Verification items for the finished model (mm, model axes). Round coordinates to 2 decimals unless told otherwise and drop trailing zeros. Order: outer loops, then holes, each group sorted by start corner. A loop starts at its lowest first (then second) coordinate and runs counter-clockwise, first axis right, second up. Notation, with made-up numbers: M 5,-21.5 L 22,-21.5 A31 cw 22,7.5 Z; hole C 56,27 d9. An arc over 180 degrees is marked long. Use CSV: the item, a comma, the result in double quotes. Start each with the question number.
Q1. Scan lines: line 1 (Y direction, x = 59, z = 0.45); line 2 (Y direction, x = 99.5, z = 0.3); line 3 (X direction, y = 33, z = 0.95). Record each from-to range of solid material in increasing order.
Q2. Sectioned sample at C-C (z = 0.65). State how many separate pieces and enclosed holes the cut face has, and give its area (3 significant figures).
Q3. Sectioned sample at A-A (x = 125). Enter the section's corners in (y, z).
Q4. Gauge pin test, flat ends, axial feed: pin 1 Ø0.5 at (x, z) = (147, 0.5) entering from +Y; pin 2 Ø2 at (x, y) = (21.21, 106.97) entering from -Z; pin 3 Ø0.5 at (x, z) = (164, 0.5) entering from +Y; pin 4 Ø0.5 at (x, z) = (102, 0.5) entering from +Y. Record the tip position at first contact, or that the pin passes through.
Q5. Sectioned sample at B-B (y = 61). Enter the section's corners in (x, z), and give its area (3 significant figures).
```python
from build123d import *
from build123d.topology import SkipClean

# Parameters (mm, degrees)
CROQUIS1_R              = 1.25
CROQUIS1_R_2            = 2.5
SALIENTE_EXTRUIR1_DEPTH = 1


with BuildPart() as part:
    # Croquis1 → Saliente-Extruir1 (new body)
    with BuildSketch(Plane.XY):
        with BuildLine():
            Line((64.278746094, 29.055249422), (61.278746094, 23.859096999))
            Line((61.278746094, 23.859096999), (67.340923921, 20.359096999))
            Line((67.340923921, 20.359096999), (85.5274574, 30.859096999))
            Line((85.5274574, 30.859096999), (112.5274574, 30.859096999))
            Line((112.5274574, 30.859096999), (112.5274574, 31.859096999))
            ThreePointArc((112.5274574, 31.859096999), (113.027457314, 32.359096999), (113.527457227, 31.859096999))
            Line((113.527457227, 31.859096999), (116.527457227, 31.859096999))
            ThreePointArc((116.527457227, 31.859096999), (117.027457227, 32.359096999), (117.527457227, 31.859096999))
            Line((117.527457227, 31.859096999), (117.527457227, 30.859096999))
            Line((117.527457227, 30.859096999), (144.527457227, 30.859096999))
            Line((144.527457227, 30.859096999), (162.713990707, 20.359096999))
            Line((162.713990707, 20.359096999), (174.83834636, 27.359096999))
            Line((174.83834636, 27.359096999), (174.83834636, 41.359096999))
            Line((174.83834636, 41.359096999), (167.83834636, 53.483452652))
            Line((167.83834636, 53.483452652), (158.83834636, 53.483452652))
            Line((158.83834636, 53.483452652), (148.446041514, 47.483452652))
            Line((148.446041514, 47.483452652), (145.446041514, 47.483452652))
            Line((145.446041514, 47.483452652), (143.946041514, 44.88537644))
            ThreePointArc((143.946041514, 44.88537644), (143.77192137, 44.012873167), (142.92105094, 44.272871814))
            Line((142.92105094, 44.272871814), (137.724898517, 47.272871814))
            Line((137.724898517, 47.272871814), (81.724898517, 47.272871814))
            Line((81.724898517, 47.272871814), (76.528746094, 50.272871814))
            Line((76.528746094, 50.272871814), (75.278746094, 48.107808305))
            ThreePointArc((75.278746094, 48.107808305), (76.193809604, 44.692744795), (72.778746094, 43.777681286))
            Line((72.778746094, 43.777681286), (71.778746094, 42.045630478))
            Line((71.778746094, 42.045630478), (72.428265147, 41.670630478))
            Line((72.428265147, 41.670630478), (64.928265147, 28.680249422))
            Line((64.928265147, 28.680249422), (64.278746094, 29.055249422))
        make_face()
        with Locations((76.571886424, 30.884748108)):
            Circle(CROQUIS1_R, mode=Mode.SUBTRACT)
        with Locations((153.286799356, 30.709365751)):
            Circle(CROQUIS1_R, mode=Mode.SUBTRACT)
        Polygon((166.425687586, 29.430249422), (165.776168533, 29.055249422), (165.12664948, 28.680249422), (157.62664948, 41.670630478), (158.276168533, 42.045630478), (158.925687586, 42.420630478), align=None, mode=Mode.SUBTRACT)
        Polygon((88.277457227, 42.272871814), (89.277457227, 43.272871814), (110.277457227, 43.272871814), (111.277457227, 42.272871814), (111.277457227, 37.272871814), (110.277457227, 36.272871814), (89.277457227, 36.272871814), (88.277457227, 37.272871814), align=None, mode=Mode.SUBTRACT)
        Polygon((119.277457227, 42.272871814), (120.277457227, 43.272871814), (133.277457227, 43.272871814), (134.277457227, 42.272871814), (134.277457227, 37.272871814), (133.277457227, 36.272871814), (120.277457227, 36.272871814), (119.277457227, 37.272871814), align=None, mode=Mode.SUBTRACT)
        with Locations((139.527457227, 41.32468677)):
            Circle(CROQUIS1_R, mode=Mode.SUBTRACT)
        with Locations((170.58834636, 40.698418571)):
            Circle(CROQUIS1_R, mode=Mode.SUBTRACT)
        with Locations((156.026168533, 45.942744795)):
            Circle(CROQUIS1_R_2, mode=Mode.SUBTRACT)
    saliente_extruir1 = extrude(amount=SALIENTE_EXTRUIR1_DEPTH)

    # Simetría2: Saliente-Extruir1 across plane
    with SkipClean():  # the faces are left unmerged after this step: merging them gives an invalid solid
        add(saliente_extruir1.mirror(Plane(origin=(35.627767514, -20.569701165, 1), x_dir=(0, 0, 1), z_dir=(0.8660254037844365, -0.5000000000000039, 0))))


solid = part.part
```
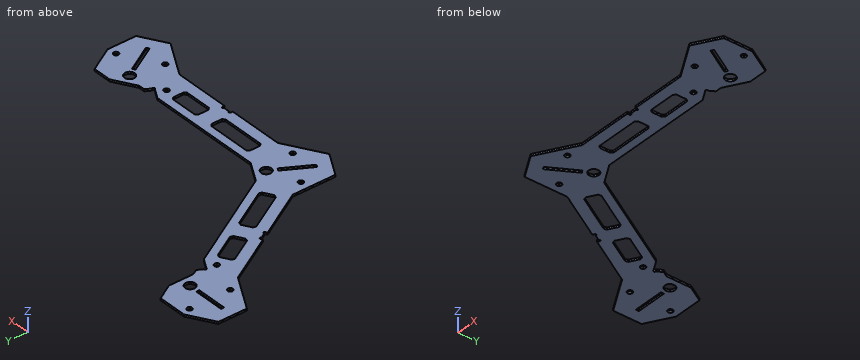
Verdict:
1,line 1,"y = 25.17 to 39.59, 41.64 to 54.05, 66.63 to 74.63"
1,line 2,"y = 30.86 to 36.27, 43.27 to 47.27"
1,line 3,"x = 55.22 to 65.69, 67.42 to 162.63, 164.36 to 174.84"
2,separate pieces,"1"
2,enclosed holes,"18"
2,area,"3,540 mm²"
3,outline,"M 30.86,0 L 36.27,0 L 36.27,1 L 30.86,1 Z; M 43.27,0 L 47.27,0 L 47.27,1 L 43.27,1 Z"
4,pin 1,"stops at y = 47.48"
4,pin 2,"passes through"
4,pin 3,"stops at y = 53.48"
4,pin 4,"stops at y = 47.27"
5,outline,"M 47.92,0 L 54.17,0 L 54.17,1 L 47.92,1 Z; M 62.25,0 L 66.87,0 L 66.87,1 L 62.25,1 Z"
5,area,"10.9 mm²"
